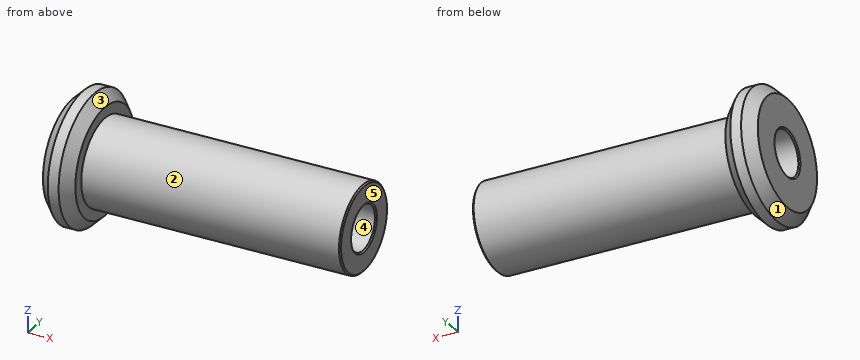
from build123d import *

# Parameters (mm, degrees)
F0_R     = 19.05
F1_DEPTH = 9.525
F2_SIZE  = 3.175
F3_R     = 12.7
F4_DEPTH = 76.2
F5_R     = 6.548438
F6_DEPTH = 85.726
F7_SIZE  = 0.396875


with BuildPart() as f1:
    # F0 (on Right) → F1 (new body)
    with BuildSketch(Plane.YZ):
        Circle(F0_R)
    extrude(amount=F1_DEPTH)

    # F2
    f2_edges = [f1.edges().sort_by_distance(p)[0] for p in [
        (9.525, -19.05, 0),
        (0, -19.05, 0),
    ]]
    chamfer(f2_edges, length=F2_SIZE)

    # F3 (on face) → F4 (join)
    with BuildSketch(Plane.YZ.offset(9.525)):
        Circle(F3_R)
    extrude(amount=F4_DEPTH)

    # F5 (on face) → F6 (cut, through all)
    with BuildSketch(Plane.YZ.offset(85.725)):
        Circle(F5_R)
    extrude(amount=-F6_DEPTH, mode=Mode.SUBTRACT)

    # F7
    f7_edges = [f1.edges().sort_by_distance(p)[0] for p in [
        (85.725, -12.7, 0),
        (85.725, -6.548438, 0),
        (0, -6.548438, 0),
    ]]
    chamfer(f7_edges, length=F7_SIZE)


solid = f1.part
Read the model definition and answer for the solid it produces. Units are mm, in the model's axes. Face numbers are marked on the shaded views. A direction names the side the tool comes from. Coordinates: 2 decimals unless noted, no trailing zeros. Write each loop counter-clockwise with the first axis right and the second up, starting at its lowest first coordinate (ties: lowest second). Pieces come first, ordered by that corner, then holes. Notation, with made-up numbers: M 53.25,39 L 106.25,39 A21 ccw 106.25,69 Z; hole C 43,89.25 d9. An arc over 180 degrees is marked long. Use a Markdown table: item, result.
Q1. The part is cut by section C-C, the plane x = 73.5. Write down the section's boundary in (y, z).
Answer block:
| item | result |
|---|---|
| outline | C 0,0 d25.4; hole C 0,0 d13.1 |
Q2. Determine the mould class of the marked faces 3, 4 and 5 for opening direction Y: released by +Y, released by -Y, zero draft, split by the parting line, or undercut.
Answer block:
| item | result |
|---|---|
| face 3 | split by the parting line |
| face 4 | undercut |
| face 5 | zero draft |
Q3. The part is cut by section A-A, the plane y = 0. Write down the section's boundary in (x, z) (3 decimals).
Answer block:
| item | result |
|---|---|
| outline | M 0,-15.875 L 3.175,-19.05 L 6.35,-19.05 L 9.525,-15.875 L 9.525,-12.7 L 85.328,-12.7 L 85.725,-12.303 L 85.725,-6.945 L 85.328,-6.548 L 0.397,-6.548 L 0,-6.945 Z; M 0,6.945 L 0.397,6.548 L 85.328,6.548 L 85.725,6.945 L 85.725,12.303 L 85.328,12.7 L 9.525,12.7 L 9.525,15.875 L 6.35,19.05 L 3.175,19.05 L 0,15.875 Z |
Q4. Straight lines are drawn through the part: L1, parallel to Z at x = 20, y = 0; L2, parallel to Y at x = 36, z = 3.5; L3, parallel to X at y = -5, z = -13.5 (3 decimals). For each, find the intervals that lie inside material, in ascending order. Write a range as [from, to].
Answer block:
| item | result |
|---|---|
| L1 | z = [-12.7, -6.55], [6.55, 12.7] |
| L2 | y = [-12.21, -5.53], [5.53, 12.21] |
| L3 | x = [0, 9.525] |
Q5. Each of these flat-tipped pins is pushed along its axis until it touches: pin 1 Ø10 at (x, y) = (59.5, -8.5) entering from +Z; pin 2 Ø2 at (x, y) = (25, -10.5) entering from -Z; pin 3 Ø2 at (x, y) = (40.5, 9) entering from -Z. Where does it stop, or does it pass through?
Answer block:
| item | result |
|---|---|
| pin 1 | stops at z = 12.21 |
| pin 2 | stops at z = -8.43 |
| pin 3 | stops at z = -9.86 |
Q6. Which of the six approach directions +Z, -Z, +X, -X, +Y, -Y give full straight-line access (tool end or side, diameter ignored) to the marked faces 1 and 2?
Answer block:
| item | result |
|---|---|
| face 1 | -X |
| face 2 | +X |
